Autodesk Inventor part; units mm, degrees
ref_plane "YZ Plane" through (0, 0, 0) normal (1, 0, 0) x (0, 1, 0)
ref_plane "XY Plane" through (0, 0, 0) normal (0, 0, 1) x (1, 0, 0)
sketch "Эскиз1" plane through (0, 0, 0) normal (0, 1, 0) x (-1, 0, 0)
  arc A0 (37, 0) -> (-37, 0) centre (0, 0) ccw
  line L0 (37, 0) -> (-37, 0)
  dimension "d0" = 37
revolve "Вращение1" add sketch "Эскиз1" angle 360 about axis through (-37, 0, 0) along (1, 0, 0)
ref_plane "РабПлоскость2" through (0, 7, 0) normal (0, 1, 0) x (-1, 0, 0)
ref_plane "РабПлоскость1" through (0, 37, 0) normal (0, 1, 0) x (-1, 0, 0)
sketch "Эскиз3" plane through (0, 0, 0) normal (1, 0, 0) x (0, 1, 0)
  circle A0 centre (0, 0) radius 37
  line L0 (6.4, -36.4423) -> (6.4, -33.4423)
  line L1 (7.6, -36.211) -> (7.6, -33.4423)
  line L2 (6.4, -33.4423) -> (7.6, -33.4423)
  line L3 (7, 51.8) -> (7, -51.8)
  point P0 (7, -33.4423)
  dimension "d3" = 3
  dimension "d4" = 1.2
sketch "Эскиз4" plane through (0, 7, 0) normal (0, 1, 0) x (-1, 0, 0)
  circle A0 centre (0, 0) radius 37.054
extrude "Выдавливание1" cut sketch "Эскиз4" against normal blind 54.75
sketch "Эскиз5" plane through (0, 7, 0) normal (0, 1, 0) x (-1, 0, 0)
  line L0 (-51.001, -36.3535) -> (49.7571, -36.3535)
  line L1 (49.7571, -36.3535) -> (49.7571, 58.6465)
  line L2 (49.7571, 58.6465) -> (-51.001, 58.6465)
  line L3 (-51.001, 58.6465) -> (-51.001, -36.3535)
  point P0 (0, 0)
  dimension "d9" = 95
extrude "Выдавливание2" add sketch "Эскиз5" against normal blind 12
properties part number "ball_2"
Input: part model. Units: mm. Frame: model coordinates. Round coordinates to 2 decimals unless told otherwise and drop trailing zeros. Write each loop counter-clockwise with the first axis right and the second up, starting at its lowest first coordinate (ties: lowest second). Pieces come first, ordered by that corner, then holes.
1) Cut plane A-A (x = -19). Return the cut outline in (y, z), then the cut area to 3 significant figures.
2) Cut plane D-D (z = 48). Return the cut outline in (x, y).
3) Cut plane C-C (y = 16.5). Return the cut outline in (x, z).
4) Ray query, L1, parallel to Y at x = -42, z = 38; L2, parallel to Z at x = 26.5, y = 9; L3, parallel to Y at x = -13, z = 27.5. Return the intervals inside material, ascending.
5) Cut plane B-B (z = 33). Return the cut outline in (x, y), then the cut area to 3 significant figures.
6) Contact query for flat-ended pins moving along their axis: P1, Ø1.5, axis at x = 15, y = 29, coming from the -Z side; P2, Ø1, axis at y = 10.5, z = -1.5, coming from the +X side; P3, Ø4, axis at x = -15, y = 25.5, coming from the -Z side. Output: stop coordinate, or through.
Geometry says:
1. outline: (-5, -36.35) - (7, -36.35) - (7, -30.97) arc R31.75 ccw to (7, 30.97) - (7, 58.65) - (-5, 58.65) - close
1. area: 2,280 mm2
2. outline: (-49.76, -5) - (51, -5) - (51, 7) - (-49.76, 7) - close
3. outline: circle Ø66.23 at (0, 0)
4. L1: y = -5 to 7
4. L2: z = -24.2 to 24.2
4. L3: y = -5 to 21.07
5. outline: (-49.76, -5) - (51, -5) - (51, 7) - (15.2, 7) arc R16.73 ccw to (-15.2, 7) - (-49.76, 7) - close
5. area: 1,420 mm2
6. P1: stops at z = -18.75
6. P2: stops at x = 35.59
6. P3: stops at z = -24.66
